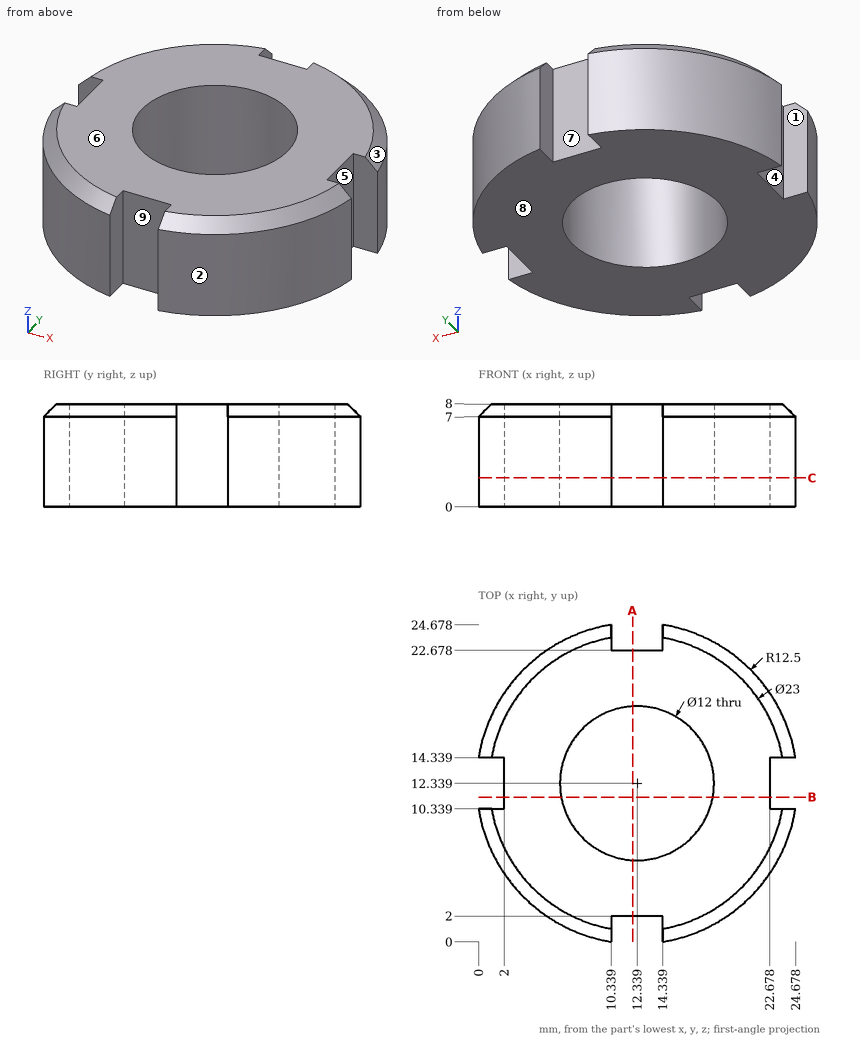
Geometry: see drawing. Coordinates: mm, zero at the bounding-box minimum. A direction names the side the tool comes from. Give positions to 0.01 mm unless a question says otherwise; leave off trailing zeros. Order: outer loops, then holes, each group sorted by start corner. A loop starts at its lowest first (then second) coordinate and runs counter-clockwise, first axis right, second up. Notation, with made-up numbers: (19, 19) - (61, 19) arc R20 ccw to (61, 55) - close; hole circle Ø1 at (40, 47). An arc over 180 degrees is marked (long way). Use a Markdown table: item, result.
(1) Draft query along Y for the marked faces 1, 2, 3 and 4. Return one class per face: released by +Y, released by -Y, zero draft, split by the parting line, or undercut.
Computed values:
| item | result |
|---|---|
| face 1 | undercut |
| face 2 | released by -Y |
| face 3 | released by +Y |
| face 4 | undercut |
(2) Access query for the marked faces 5, 6, 7, 8 and 9. Directions: +Z, -Z, +X, -X, +Y, -Y. A direction counts if a zero-diameter tool reaches every point of the face in a straight line with its end or side. Return the directions, or none.
Computed values:
| item | result |
|---|---|
| face 5 | +Z, -Z, +X |
| face 6 | +Z, +X, -X, +Y, -Y |
| face 7 | +Z, -Z, +Y |
| face 8 | -Z, +X, -X, +Y, -Y |
| face 9 | +Z, -Z, -Y |
(3) Section query B-B (y = 11.25). Output: boundary loops of the cut face in (x, z).
Computed values:
| item | result |
|---|---|
| outline | (2, 0) - (6.44, 0) - (6.44, 8) - (2, 8) - close; (18.24, 0) - (22.68, 0) - (22.68, 8) - (18.24, 8) - close |
(4) Section query C-C (z = 2.25). Output: boundary loops of the cut face in (x, y), then the cut area to 3 significant figures.
Computed values:
| item | result |
|---|---|
| outline | (0, 10.34) arc R12.5 ccw to (10.34, 0) - (10.34, 2) - (14.34, 2) - (14.34, 0) arc R12.5 ccw to (24.68, 10.34) - (22.68, 10.34) - (22.68, 14.34) - (24.68, 14.34) arc R12.5 ccw to (14.34, 24.68) - (14.34, 22.68) - (10.34, 22.68) - (10.34, 24.68) arc R12.5 ccw to (0, 14.34) - (2, 14.34) - (2, 10.34) - close; hole circle Ø12 at (12.34, 12.34) |
| area | 344 mm2 |
(5) Line query: line 1 (Y direction, x = 13, z = 6); line 2 (Y direction, x = 14.75, z = 2); line 3 (X direction, y = 7.5, z = 4.75). Output: solid intervals per line, ascending. Write a range as from..to.
Computed values:
| item | result |
|---|---|
| line 1 | y = 2..6.38, 18.3..22.68 |
| line 2 | y = 0.07..6.84, 17.83..24.6 |
| line 3 | x = 0.81..8.79, 15.89..23.86 |
(6) Pin query (flat end, axial travel): pin 1 (1 mm diameter, centred on x = 23.5, z = 5.5, fed in from +Y) (1 decimal); pin 2 (2 mm diameter, centred on x = 24, z = 2, fed in from -Y); pin 3 (0.6 mm diameter, centred on y = 1, z = 2, fed in from +X); pin 4 (7 mm diameter, centred on x = 12.34, y = 12.34, fed in from -Z). Return the tip coordinate at first contact, or that it passes through.
Computed values:
| item | result |
|---|---|
| pin 1 | stops at y = 18.9 |
| pin 2 | stops at y = 5.81 |
| pin 3 | stops at x = 18.2 |
| pin 4 | passes through |
(7) Section query A-A (x = 12). Output: boundary loops of the cut face in (y, z).
Computed values:
| item | result |
|---|---|
| outline | (2, 0) - (6.35, 0) - (6.35, 8) - (2, 8) - close; (18.33, 0) - (22.68, 0) - (22.68, 8) - (18.33, 8) - close |
